The model under review builds one solid part; all positions refer to its coordinate system, in mm. A direction names the side the tool comes from. Round coordinates to 2 decimals unless told otherwise and drop trailing zeros. Write each loop counter-clockwise with the first axis right and the second up, starting at its lowest first coordinate (ties: lowest second). Pieces come first, ordered by that corner, then holes. Notation, with made-up numbers: (74, -32) -> (99, -32) arc R30 cw to (99, 2) -> close; hole circle Ø9 at (51, -8.75). An arc over 180 degrees is marked (long way). Use CSV: the item, a comma, the result in double quotes. Start each with the question number.
1) Take a section at A-A, the plane z = 0. Give the boundary of the cut face in (x, y) (3 decimals), then the cut area to 3 significant figures.
2) Wall thickness on probe 1 along X at (y, z) = (105.5, 3.25); probe 2 along X at (y, z) = (16, 1); probe 3 along Z at (x, y) = (-0.5, 84.5): over which ranges is each line inside the solid? List them lowest first. Write a range as [from, to].
3) For pin 1 Ø10 at (x, y) = (4.5, 45.5) entering from +Z; pin 2 Ø10 at (x, y) = (7.5, 24.5) entering from +Z; pin 3 Ø2 at (y, z) = (55.5, 10.5) entering from -X; pin 4 Ø9 at (x, z) = (0, 0) entering from +Y, all flat-tipped, find the tip position at first contact; note any pin that passes through.
4) Take a section at D-D, the plane y = 8. Give the boundary of the cut face in (x, z) (3 decimals).
5) Take a section at C-C, the plane y = 83. Give the boundary of the cut face in (x, z) (3 decimals).
6) Mouldability with a two-part tool opening along Z and no side actions: class faces 3 (the face through (-6, 0, 6)), 4 (the face through (-13.67, 1.48, -3.03)), 5 (the face through (-7.346, 62.361, -1.631)) as released by +Z, released by -Z, zero draft, split by the parting line, or undercut.
7) Machinability: for faces 1 (the face through (-7.23, 123, -2.62)), 2 (the face through (-3.77, 62.16, -11.98)), which of the approach directions +Z, -Z, +X, -X, +Y, -Y give a long, thin tool a straight path to every point of the face, cutting with its end or side? Answer none if there is none.
8) Take a section at B-B, the plane x = 0. Give the boundary of the cut face in (y, z) (3 decimals), then the cut area to 3 significant figures.
from build123d import *

# Parameters (mm, degrees)
CROQUIS1_R              = 14
SALIENTE_EXTRUIR1_DEPTH = 3
CROQUIS2_R              = 11.075
SALIENTE_EXTRUIR2_DEPTH = 120
CROQUIS3_R              = 7.525
CORTAR_EXTRUIR2_DEPTH   = 125.583305463


with BuildPart() as part:
    # Croquis1 → Saliente-Extruir1 (new body)
    with BuildSketch(Plane(origin=(0, 0, 0), x_dir=(1, 0, 0), z_dir=(0, 1, 0))):
        with Locations(Location((0, 0, 0), (0, 0, 270))):
            Circle(CROQUIS1_R)
    extrude(amount=SALIENTE_EXTRUIR1_DEPTH)

    # Croquis2 → Saliente-Extruir2 (add)
    with BuildSketch(Plane(origin=(0, 3, 0), x_dir=(1, 0, 0), z_dir=(0, 1, 0))):
        with Locations(Location((0, 0, 0), (0, 0, 270))):
            Circle(CROQUIS2_R)
    extrude(amount=SALIENTE_EXTRUIR2_DEPTH)

    # Croquis3 → Cortar-Extruir2 (cut, through all)
    with BuildSketch(Plane(origin=(0, 123, 0), x_dir=(1, 0, 0), z_dir=(0, 1, 0))):
        with Locations(Location((0, 0, 0), (0, 0, 270))):
            Circle(CROQUIS3_R)
    extrude(amount=-CORTAR_EXTRUIR2_DEPTH, mode=Mode.SUBTRACT)

    # Croquis4 → Revolución1 (revolve)
    with BuildSketch(Plane.XY, mode=Mode.PRIVATE) as revoluci_n1_sk:
        Polygon((14, 3), (11.075, 3), (11.075, 123), align=None)
    revolve(revoluci_n1_sk.sketch.rotate(Axis((0, 0, 0), (0, 1, 0)), 90), axis=Axis((0, 0, 0), (0, 1, 0)))


solid = part.part
Values found:
1,outline,"(-14, 0) -> (-7.525, 0) -> (-7.525, 123) -> (-11.075, 123) -> (-14, 3) -> close; (7.525, 0) -> (14, 0) -> (14, 3) -> (11.075, 123) -> (7.525, 123) -> close"
1,area,"1,240 mm²"
2,probe 1,"[-11.03, -6.79], [6.79, 11.03]"
2,probe 2,"[-13.65, -7.46], [7.46, 13.65]"
2,probe 3,"[-12, -7.51], [7.51, 12]"
3,pin 1,"z = 13.03"
3,pin 2,"z = 13.25"
3,pin 3,"x = -8.46"
3,pin 4,"through"
4,outline,"circle Ø27.756 at (0, 0); hole circle Ø15.05 at (0, 0)"
5,outline,"circle Ø24.1 at (0, 0); hole circle Ø15.05 at (0, 0)"
6,face 3,"zero draft"
6,face 4,"split by the parting line"
6,face 5,"undercut"
7,face 1,"+Z, -Z, +X, -X, +Y"
7,face 2,"+Y"
8,outline,"(0, -14) -> (3, -14) -> (123, -11.075) -> (123, -7.525) -> (0, -7.525) -> close; (0, 7.525) -> (123, 7.525) -> (123, 11.075) -> (3, 14) -> (0, 14) -> close"
8,area,"1,240 mm²"
